Can you work these out from the model? Positions are in its coordinate system, mm. Face numbers are marked on the shaded views. Round coordinates to 2 decimals unless told otherwise and drop trailing zeros. Loops run counter-clockwise (first coordinate to the right, second up) from the corner with the lowest first, then second, coordinate; pieces in that order, holes last. Notation, with made-up numbers: (68.25, 52) -> (72.25, 52) arc R24 cw to (72.25, 69) -> close; hole circle Ø2 at (15.5, 60.25). An arc over 180 degrees is marked (long way). Use a Markdown table: item, result.
Autodesk Inventor part; units mm, degrees
ref_plane "作業平面1" through (0, 6, 0) normal (0, 1, 0) x (-1, 0, 0)
ref_plane "YZ Plane" through (0, 0, 0) normal (1, 0, 0) x (0, 1, 0)
ref_plane "XY Plane" through (0, 0, 0) normal (0, 0, 1) x (1, 0, 0)
sketch "スケッチ1" plane through (0, 0, 0) normal (0, 0, 1) x (1, 0, 0)
  circle A0 centre (0, 0) radius 6
  dimension "d0" = 12
extrude "押し出し1" add sketch "スケッチ1" along normal blind 59
ref_plane "作業平面1" through (0, 6, 0) normal (0, 1, 0) x (-1, 0, 0)
sketch "スケッチ2" plane through (0, 6, 0) normal (0, 1, 0) x (-1, 0, 0)
  line L0 (0, 0) -> (2, 0)
  line L1 (2, 0) -> (2, 20)
  line L2 (2, 20) -> (0, 20)
  line L3 (0, 20) -> (0, 0)
  line L4 (6, 0) -> (-6, 0)
  line L5 (0, 20) -> (-2, 20)
  line L6 (-2, 20) -> (-2, 0)
  line L7 (-2, 0) -> (0, 0)
  line L8 (0, 0) -> (0, 20)
  dimension "d3" = 2
  dimension "d4" = 20
  dimension "d5" = 2
extrude "押し出し2" cut sketch "スケッチ2" against normal blind 6
sketch "スケッチ3" plane through (0, 0, 0) normal (0, 0, -1) x (-1, 0, 0)
  point P0 (0, 0)
  point P1 (0, 0)
hole "穴1" at (0, 0, 0) direction (0, 0, 1) diameter 8 depth 20 tip angle 118
sketch "スケッチ4" plane through (0, 6, 0) normal (0, 1, 0) x (-1, 0, 0)
  line L0 (2, 20) -> (-2, 20)
  point P0 (0, 0)
  point P1 (0, 45)
  dimension "d15" = 25
hole "穴2" at (0, 6, 45) direction (0, -1, 0) diameter 4 end through all
sketch "スケッチ5" plane through (0, 6, 0) normal (0, 1, 0) x (-1, 0, 0)
  line L0 (6, 59) -> (-6, 59)
  point P0 (0, 0)
  point P1 (0, 56)
  dimension "d23" = 3
hole "穴3" at (0, 6, 56) direction (0, -1, 0) diameter 2 end through all
properties part number "TH22_Bar_motor_roller_sn" material "アルミニウム 6061-AHC"
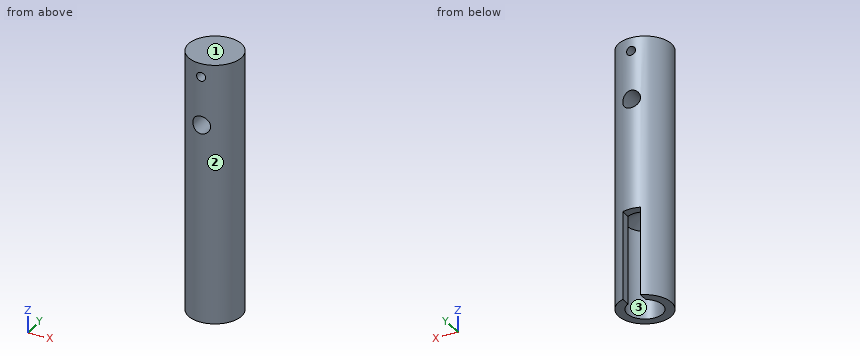
1. I want a section at C-C (z = 35.5). Please give me the cut outline in (x, y).
Answer sheet:
| item | result |
|---|---|
| outline | circle Ø12 at (0, 0) |
2. If we mould it in two halves opening along Y, with no side actions, what happens to the marked faces 1, 2 and 3? For each: +Y half, -Y half, draft (parallel to the pull), parting line (faces both ways), or undercut.
Answer sheet:
| item | result |
|---|---|
| face 1 | draft |
| face 2 | parting line |
| face 3 | undercut |
3. Will these pins go through, and if not, where does the flat tip stop? pin 1 Ø2 at (y, z) = (3.5, 25) entering from +X; pin 2 Ø1.8 at (y, z) = (5, 13) entering from -X; pin 3 Ø1.5 at (x, z) = (-4.5, 47) entering from -Y.
Answer sheet:
| item | result |
|---|---|
| pin 1 | stops at x = 5.45 |
| pin 2 | stops at x = -4.38 |
| pin 3 | stops at y = -4.68 |
4. I want a section at A-A (z = 56). Please give me the cut outline in (x, y).
Answer sheet:
| item | result |
|---|---|
| outline | (-1, -5.92) -> (-1, 5.92) arc R6 ccw to start; (1, -5.92) arc R6 ccw to (1, 5.92) -> close |
5. I want a section at B-B (y = -3.25). State how many separate pieces and enclosed holes the cut face has, plus the area to 3 significant figures.
Answer sheet:
| item | result |
|---|---|
| separate pieces | 1 |
| enclosed holes | 2 |
| area | 485 mm² |
6. I need wall thicknesses on line 1 (Z direction, x = -0.25, y = 5.5); line 2 (X direction, y = 2.75, z = 16); line 3 (X direction, y = -2.5, z = 45). Which ranges of each line are inside material? Lowest first, please.
Answer sheet:
| item | result |
|---|---|
| line 1 | z = 20 to 43.02, 46.98 to 55.03, 56.97 to 59 |
| line 2 | x = -5.33 to -2.9, 2.9 to 5.33 |
| line 3 | x = -5.45 to -2, 2 to 5.45 |
